Geometry check sheet. Reference: the model listing, model coordinates, mm. Face numbers are marked on the shaded views. A direction names the side the tool comes from. Give positions to 0.01 mm unless a question says otherwise; leave off trailing zeros. Write each loop counter-clockwise with the first axis right and the second up, starting at its lowest first coordinate (ties: lowest second). Pieces come first, ordered by that corner, then holes. Notation, with made-up numbers: M 37.25,-7 L 54.25,-7 A21 ccw 54.25,-3 Z; hole C 49,53.25 d5. An arc over 180 degrees is marked long. One line per item, written item: value. Start each with the question number.
1. Gauge pin test, flat ends, axial feed: pin 1 (3 mm diameter, centred on x = -40.5, z = -9.5, fed in from +Y); pin 2 (8 mm diameter, centred on x = -20.5, y = 3, fed in from -Z); pin 3 (5 mm diameter, centred on y = 9, z = 7.5, fed in from +X). Record the tip position at first contact, or that the pin passes through.
2. Cross-section at D-D on y = 5.75. Record the cut outline in (x, z).
3. Cross-section at A-A on y = 0. Record the cut outline in (x, z).
4. Tool access check on the marked faces 1, 2 and 3. Record the directions out of +Z, -Z, +X, -X, +Y, -Y that give a thin tool (end or side, any length) a straight path to the whole face; none if there is none.
5. Scan lines: line 1 (Y direction, x = -1.9, z = 0); line 2 (X direction, y = 2, z = 6.5); line 3 (Z direction, x = -1.25, y = 8.5). Record each from-to range of solid material in increasing order.
6. Cross-section at C-C on x = -29. Record the cut outline in (y, z), then the cut area to 3 significant figures.
7. Cross-section at B-B on z = 6. Record the cut outline in (x, y).
from build123d import *

# Parameters (mm, degrees)
SKETCH2_R               = 12.5
BOSS_EXTRUDE1_DEPTH     = 17
SKETCH3_R               = 12.2
BOSS_EXTRUDE2_DEPTH     = 30.8
SKETCH4_R               = 3.5
BOSS_EXTRUDE3_DEPTH     = 2.5
SKETCH5_R               = 2
BOSS_EXTRUDE4_DEPTH     = 10
CUT_EXTRUDE1_DEPTH      = 63.837807091
CUT_EXTRUDE1_DEPTH_BACK = 8
M3_TAPPED_HOLE1_D       = 2.5
M3_TAPPED_HOLE1_DEPTH   = 4.55
M3_TAPPED_HOLE1_TIP     = 0.751075774


with BuildPart() as part:
    # Sketch2 → Boss-Extrude1 (new body)
    with BuildSketch(Plane(origin=(0, 0, 0), x_dir=(0, 0, -1), z_dir=(1, 0, 0))):
        Circle(SKETCH2_R)
    extrude(amount=-BOSS_EXTRUDE1_DEPTH)

    # Sketch3 → Boss-Extrude2 (add)
    with BuildSketch(Plane.ZY.offset(17)):
        with Locations(Location((0, 0, 0), (0, 0, 180))):
            Circle(SKETCH3_R)
    extrude(amount=BOSS_EXTRUDE2_DEPTH)

    # Sketch4 → Boss-Extrude3 (add)
    with BuildSketch(Plane(origin=(0, 0, 0), x_dir=(0, 0, -1), z_dir=(1, 0, 0))):
        Circle(SKETCH4_R)
    extrude(amount=BOSS_EXTRUDE3_DEPTH)

    # Sketch5 → Boss-Extrude4 (add)
    with BuildSketch(Plane(origin=(2.5, 0, 0), x_dir=(0, 0, -1), z_dir=(1, 0, 0))):
        Circle(SKETCH5_R)
    extrude(amount=BOSS_EXTRUDE4_DEPTH)

    # Sketch6 → Cut-Extrude1 (cut, two sides: drawn at the far end of the back side and taken through both)
    with BuildSketch(Plane(origin=(12.5, 0, 0), x_dir=(0, 0, -1), z_dir=(1, 0, 0)).offset(-CUT_EXTRUDE1_DEPTH_BACK)):
        Polygon((-50.671161076, 1.5), (-1.322875656, 1.5), (1.322875656, 1.5), (50.671161076, 1.5), (50.671161076, 100.196570842), (-50.671161076, 100.196570842), align=None)
    extrude(amount=CUT_EXTRUDE1_DEPTH + CUT_EXTRUDE1_DEPTH_BACK, mode=Mode.SUBTRACT)

    # M3 Tapped Hole1
    with Locations(Plane(origin=(0, 0, 0), x_dir=(0, 0, -1), z_dir=(1, 0, 0))):
        with Locations((0, 8.5), (0, -8.5)):
            Hole(M3_TAPPED_HOLE1_D / 2, depth=M3_TAPPED_HOLE1_DEPTH)
            with Locations((0, 0, -(M3_TAPPED_HOLE1_DEPTH + M3_TAPPED_HOLE1_TIP / 2))):  # 118° drill point
                Cone(0, M3_TAPPED_HOLE1_D / 2, M3_TAPPED_HOLE1_TIP, mode=Mode.SUBTRACT)


solid = part.part
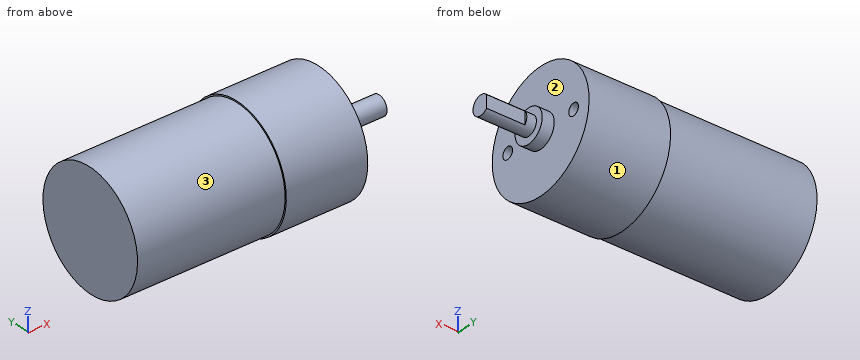
Report:
1. pin 1: stops at y = 9.21
1. pin 2: stops at z = -12.45
1. pin 3: stops at x = 0
2. outline: M -47.8,-10.76 L -17,-10.76 L -17,-11.1 L 0,-11.1 L 0,11.1 L -17,11.1 L -17,10.76 L -47.8,10.76 Z
3. outline: M -47.8,-12.2 L -17,-12.2 L -17,-12.5 L 0,-12.5 L 0,-3.5 L 2.5,-3.5 L 2.5,-2 L 12.5,-2 L 12.5,2 L 2.5,2 L 2.5,3.5 L 0,3.5 L 0,12.5 L -17,12.5 L -17,12.2 L -47.8,12.2 Z
4. face 1: +X, -X
4. face 2: +X
4. face 3: -X
5. line 1: y = -12.5 to -9.75, -7.25 to 7.25, 9.75 to 12.5
5. line 2: x = -47.8 to 0
5. line 3: z = -9.17 to -1.25, 1.25 to 9.17
6. outline: C 0,0 d24.4
6. area: 468 mm^2
7. outline: M -47.8,-10.62 L -17,-10.62 L -17,-10.97 L 0,-10.97 L 0,10.97 L -17,10.97 L -17,10.62 L -47.8,10.62 Z
